from build123d import *

# Parameters (mm, degrees)
SKETCH1_R           = 37
BOSS_EXTRUDE1_DEPTH = 5
CUT_EXTRUDE3_START  = -10
CUT_EXTRUDE3_DEPTH  = 10
FILLET2_R           = 25
FILLET3_R           = 20
SKETCH7_W           = 5
SKETCH7_H           = 5
SKETCH7_W_2         = 7
CUT_EXTRUDE4_DEPTH  = 10


with BuildPart() as part:
    # Sketch1 → Boss-Extrude1 (new body)
    with BuildSketch(Plane.XY):
        Circle(SKETCH1_R)
    extrude(amount=BOSS_EXTRUDE1_DEPTH)

    # Sketch6 → Cut-Extrude3 (cut)
    with BuildSketch(Plane.XY.offset(5).offset(CUT_EXTRUDE3_START)):
        with BuildLine():
            Line((-25, 27.276363394), (-25, -27.276363394))
            ThreePointArc((-25, -27.276363394), (-37, 0), (-25, 27.276363394))
        make_face()
        with BuildLine():
            Line((25, -27.276363394), (25, 27.276363394))
            ThreePointArc((25, 27.276363394), (37, 0), (25, -27.276363394))
        make_face()
    extrude(amount=CUT_EXTRUDE3_DEPTH, mode=Mode.SUBTRACT)

    # Fillet2
    fillet2_edges = [part.edges().sort_by_distance(p)[0] for p in [
        (-25, 27.276363394, 2.5),
        (25, 27.276363394, 2.5),
    ]]
    fillet(fillet2_edges, radius=FILLET2_R - 0.0001)  # a hair under: the kernel refuses the full size

    # Fillet3
    fillet3_edges = [part.edges().sort_by_distance(p)[0] for p in [
        (-25, -27.276363394, 2.5),
        (25, -27.276363394, 2.5),
    ]]
    fillet(fillet3_edges, radius=FILLET3_R)

    # Sketch7 → Cut-Extrude4 (cut)
    with BuildSketch(Plane.XY.offset(5)):
        with Locations((0, 24)):
            Rectangle(SKETCH7_W, SKETCH7_H)
        with Locations((0, -23.5)):
            Rectangle(SKETCH7_W_2, SKETCH7_H)
    extrude(amount=-CUT_EXTRUDE4_DEPTH, mode=Mode.SUBTRACT)


solid = part.part
Geometry check sheet. Reference: the model listing, model coordinates, mm. A direction names the side the tool comes from. Coordinates: 2 decimals unless noted, no trailing zeros. Write each loop counter-clockwise with the first axis right and the second up, starting at its lowest first coordinate (ties: lowest second). Pieces come first, ordered by that corner, then holes. Notation, with made-up numbers: (77.25, 37) -> (136.25, 37) arc R21 cw to (136.25, 70) -> close; hole circle Ø3 at (3, -3). An arc over 180 degrees is marked (long way). One line per question, with ' | ' between items.
1. Cross-section at D-D on x = -13.5. Record the cut outline in (y, z), and give its area (3 significant figures).
Answers:
outline: (-34.35, 0) -> (33.04, 0) -> (33.04, 5) -> (-34.35, 5) -> close | area: 337 mm²
2. Draft check along Y on faces 1 (the flat face through (-25, -2, 2)), 2 (the cylindrical face through (0, -37, 2)), 3 (the flat face through (-2.5, 24, 3)). Enter one of: +Y half, -Y half, draft (parallel to the pull), parting line (faces both ways), or undercut.
Answers:
face 1: draft | face 2: -Y half | face 3: undercut
3. Cross-section at B-B on z = 3.45. State how many separate pieces and enclosed holes the cut face has, and give its area (3 significant figures).
Answers:
separate pieces: 1 | enclosed holes: 2 | area: 3,170 mm²
4. Cross-section at A-A on x = 1.5. Record the cut outline in (y, z).
Answers:
outline: (-36.97, 0) -> (-26, 0) -> (-26, 5) -> (-36.97, 5) -> close; (-21, 0) -> (21.5, 0) -> (21.5, 5) -> (-21, 5) -> close; (26.5, 0) -> (36.95, 0) -> (36.95, 5) -> (26.5, 5) -> close
5. Thickness scan on probe 1 along Y at (x, z) = (-1, 4.7); probe 2 along X at (y, z) = (34.5, 1.55); probe 3 along X at (y, z) = (23, 1.65). Record the ranges inside material, lowest first. Write a range as from..to.
Answers:
probe 1: y = -36.99..-26, -21..21.5, 26.5..36.98 | probe 2: x = -10.9..10.9 | probe 3: x = -22.45..-2.5, 2.5..22.45
6. Depth check by flat-ended pin: pin 1 Ø2.5 at (y, z) = (25, 2) entering from -X; pin 2 Ø8 at (x, y) = (15, -12.5) entering from -Z; pin 3 Ø2 at (x, z) = (-9.5, 2) entering from -Y; pin 4 Ø1 at (x, z) = (-12.5, 4) entering from +Y. Enter the tip coordinate at first touch or a pass-through.
Answers:
pin 1: stops at x = -22.07 | pin 2: stops at z = 0 | pin 3: stops at y = -36.01 | pin 4: stops at y = 33.93
7. Set-up check for faces 4 (the flat face through (0, 1, 0)), 5 (the flat face through (0, 26.5, 3)): record each of +Z, -Z, +X, -X, +Y, -Y from which the full face is reachable in a straight line by a thin tool's end or side.
Answers:
face 4: -Z, +X, -X, +Y, -Y | face 5: +Z, -Z
8. Cross-section at C-C on y = -30.5. Record the cut outline in (x, z).
Answers:
outline: (-19.03, 0) -> (19.03, 0) -> (19.03, 5) -> (-19.03, 5) -> close
